Model file for the job. Use its own axes, mm. A direction names the side the tool comes from. Coordinates: 2 decimals unless noted, no trailing zeros. Write each loop counter-clockwise with the first axis right and the second up, starting at its lowest first coordinate (ties: lowest second). Pieces come first, ordered by that corner, then holes. Notation, with made-up numbers: M 66.25,55.25 L 120.25,55.25 A14 ccw 120.25,72.25 Z; hole C 38,16.5 d6. An arc over 180 degrees is marked long. Put each result on its own line as item: value. Start each with the question number.
Q1. Cut at C-C (z = 4). Write the cut outline in (x, y) (3 decimals), then the cut area to 3 significant figures.
Q2. Cut at B-B (x = 4.5). Write the cut outline in (y, z) (1 decimal), then the cut area to 3 significant figures.
Q3. Pull direction Z, two halves, no side cores. Call faces 1 (the flat face through (0, 2, -18.351)), 2 (the flat face through (-18, 2, -12.636)), 3 (the flat face through (0, 2, 15.176)): pulls with the +Z half, pulls with the -Z half, needs draft (parallel to the pull), parting line crosses it, or undercut.
Q4. Cut at D-D (y = 1). Give the number of separate pieces and of enclosed holes in the cut face, then the cut area to 3 significant figures.
Q5. Drop a flat-ended pin along its axis: pin 1 (2.5 mm diameter, centred on x = 25.59, z = 4.76, fed in from -Y) (3 decimals). Give the stop position or say it passes through.
Q6. Drill centre lines: line 1 along Z through (x, y) = (-18.5, 2.35); line 2 along X through (y, z) = (2.1, -13.5); line 3 along Z through (x, y) = (21.5, 2.6). Where is each one in solid material? Low to high.
Q7. Which spindle directions (+Z, -Z, +X, -X, +Y, -Y) get a long thin tool onto all of the face, cutting with end or side? Do faces 4 (the flat face through (-8, 3.175, -13)), 5 (the flat face through (0, 2, 10.096)). Say none if no direction does.
Q8. Cut at A-A (x = 14.5). Write the cut outline in (y, z) (1 decimal).
```python
from build123d import *

# Parameters (mm, degrees)
SKETCH1_W           = 65.786
SKETCH1_H           = 33.528
SKETCH1_R           = 2.2225
SKETCH1_W_2         = 10.16
SKETCH1_H_2         = 3.175
BOSS_EXTRUDE2_DEPTH = 3.175


with BuildPart() as part:
    # Sketch1 → Boss-Extrude2 (new body)
    with BuildSketch(Plane(origin=(0, 0, 0), x_dir=(1, 0, 0), z_dir=(0, 1, 0))):
        with Locations((0, 1.5875)):
            Rectangle(SKETCH1_W, SKETCH1_H)
        with Locations(Location((-25.5905, -4.7625, 0), (0, 0, 270))):
            Circle(SKETCH1_R, mode=Mode.SUBTRACT)
        Polygon((20.701, -10.0965), (-20.701, -10.0965), (-20.701, -1.27), (-25.273, -1.27), (-25.273, 1.27), (-20.701, 1.27), (-20.701, 10.0965), (20.701, 10.0965), (20.701, 1.27), (25.273, 1.27), (25.273, -1.27), (20.701, -1.27), align=None, mode=Mode.SUBTRACT)
        with Locations(Location((25.5905, -4.7625, 0), (0, 0, 270))):
            Circle(SKETCH1_R, mode=Mode.SUBTRACT)
        with Locations(Location((-25.5905, 4.7625, 0), (0, 0, 270))):
            Circle(SKETCH1_R, mode=Mode.SUBTRACT)
        with Locations((-17.907, 14.224)):
            Rectangle(SKETCH1_W_2, SKETCH1_H_2, mode=Mode.SUBTRACT)
        with Locations(Location((25.5905, 4.7625, 0), (0, 0, 270))):
            Circle(SKETCH1_R, mode=Mode.SUBTRACT)
        with Locations((2.413, 14.224)):
            Rectangle(SKETCH1_W_2, SKETCH1_H_2, mode=Mode.SUBTRACT)
        with Locations((22.733, 14.224)):
            Rectangle(SKETCH1_W_2, SKETCH1_H_2, mode=Mode.SUBTRACT)
    extrude(amount=BOSS_EXTRUDE2_DEPTH)


solid = part.part
```
Computed values:
1. outline: M -32.893,0 L -27.678,0 L -27.678,3.175 L -32.893,3.175 Z; M -23.503,0 L -20.701,0 L -20.701,3.175 L -23.503,3.175 Z; M 20.701,0 L 23.503,0 L 23.503,3.175 L 20.701,3.175 Z; M 27.678,0 L 32.893,0 L 32.893,3.175 L 27.678,3.175 Z
1. area: 50.9 mm2
2. outline: M 0,-18.4 L 3.2,-18.4 L 3.2,-15.8 L 0,-15.8 Z; M 0,-12.6 L 3.2,-12.6 L 3.2,-10.1 L 0,-10.1 Z; M 0,10.1 L 3.2,10.1 L 3.2,15.2 L 0,15.2 Z
2. area: 32.3 mm2
3. face 1: pulls with the -Z half
3. face 2: undercut
3. face 3: pulls with the +Z half
4. separate pieces: 1
4. enclosed holes: 8
4. area: 1,190 mm2
5. pin 1: through
6. line 1: -18.35 to -15.81, -12.64 to -10.1, 10.1 to 15.18
6. line 2: -32.89 to -22.99, -12.83 to -2.67, 7.49 to 17.65, 27.81 to 32.89
6. line 3: -18.35 to -15.81, -12.64 to -1.27, 1.27 to 15.18
7. face 4: +Z, -Z, +X, -X, +Y
7. face 5: +Y, -Y
8. outline: M 0,-18.4 L 3.2,-18.4 L 3.2,-10.1 L 0,-10.1 Z; M 0,10.1 L 3.2,10.1 L 3.2,15.2 L 0,15.2 Z
